The model under review builds one solid part; all positions refer to its coordinate system, in mm. Face numbers are marked on the shaded views. Give positions to 0.01 mm unless a question says otherwise; leave off trailing zeros. Order: outer loops, then holes, each group sorted by start corner. A loop starts at its lowest first (then second) coordinate and runs counter-clockwise, first axis right, second up. Notation, with made-up numbers: (-22, 20) - (25, 20) arc R35 ccw to (25, 53) - close; hole circle Ø2 at (11.25, -16.5). An arc over 180 degrees is marked (long way). Write item = value, one per line. Start each with the question number.
1. For P1, Ø1.2, axis at x = -14.5, y = -2.5, coming from the +Z side; P2, Ø9, axis at x = 13, z = 23.5, coming from the -Y side, all flat-tipped, find the tip position at first contact; note any pin that passes through.
2. Wall thickness on probe 1 along Z at (x, y) = (0, -0.7); probe 2 along X at (y, z) = (-1, 70); probe 3 along Y at (x, z) = (-16, 47): over which ranges is each line inside the solid? List them lowest first.
3. We need section A-A, the plane z = 10. Give the boundary of the cut face in (x, y), and give its area (3 significant figures).
4. We need section B-B, the plane x = 0. Give the boundary of the cut face in (y, z), and give its area (3 significant figures).
5. We need section D-D, the plane x = 14. Give the boundary of the cut face in (y, z), and give its area (3 significant figures).
6. Mouldability with a two-part tool opening along Y and no side actions: class the marked faces 1, 2 and 3 as pulls with the +Y half, pulls with the -Y half, needs draft (parallel to the pull), parting line crosses it, or undercut.
7. We need section C-C, the plane z = 60.5. Give the boundary of the cut face in (x, y), and give its area (3 significant figures).
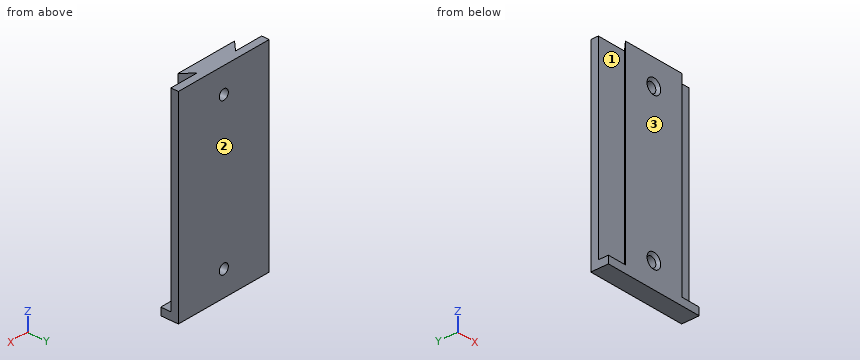
from build123d import *

# Parameters (mm, degrees)
F1_DEPTH = 80
F2_R     = 2
F3_DEPTH = 12.5
F4_SIZE  = 1
F5_W     = 40
F5_H     = 4
F6_DEPTH = 3


with BuildPart() as f1:
    # F0 (on Top) → F1 (new body)
    with BuildSketch(Plane.XY):
        Polygon((20, 1.5), (-20, 1.5), (-20, -1.5), (-8.5, -1.5), (8.5, -1.5), (20, -1.5), align=None)
        Polygon((8.5, -1.5), (-8.5, -1.5), (-12.5, -5.5), (12.5, -5.5), align=None)
    extrude(amount=F1_DEPTH)

    # F2 (on face) → F3 (cut, symmetric)
    with BuildSketch(Plane.XZ.offset(1.5)):
        with Locations((0, 70)):
            Circle(F2_R)
        with Locations((0, 10)):
            Circle(F2_R)
    extrude(amount=F3_DEPTH, both=True, mode=Mode.SUBTRACT)

    # F4
    f4_edges = [f1.edges().sort_by_distance(p)[0] for p in [
        (-2, -5.5, 70),
        (-2, -5.5, 10),
    ]]
    chamfer(f4_edges, length=F4_SIZE)

    # F5 (on Top) → F6 (join)
    with BuildSketch(Plane.XY):
        with Locations((0, -3.5)):
            Rectangle(F5_W, F5_H)
    extrude(amount=F6_DEPTH)


solid = f1.part
Model answer:
q1.P1 = 3
q1.P2 = -5.5
q2.probe_1 = 0 to 8, 12 to 68, 72 to 80
q2.probe_2 = -20 to -2, 2 to 20
q2.probe_3 = -1.5 to 1.5
q3.outline = (-20, -1.5) - (-8.5, -1.5) - (-12.5, -5.5) - (-3, -5.5) - (-2, -4.5) - (-2, 1.5) - (-20, 1.5) - close; (2, -4.5) - (3, -5.5) - (12.5, -5.5) - (8.5, -1.5) - (20, -1.5) - (20, 1.5) - (2, 1.5) - close
q3.area = 175 mm2
q4.outline = (-5.5, 0) - (1.5, 0) - (1.5, 8) - (-4.5, 8) - (-5.5, 7) - close; (-5.5, 13) - (-4.5, 12) - (1.5, 12) - (1.5, 68) - (-4.5, 68) - (-5.5, 67) - close; (-5.5, 73) - (-4.5, 72) - (1.5, 72) - (1.5, 80) - (-5.5, 80) - close
q4.area = 502 mm2
q5.outline = (-5.5, 0) - (1.5, 0) - (1.5, 80) - (-1.5, 80) - (-1.5, 3) - (-5.5, 3) - close
q5.area = 252 mm2
q6.face_1 = undercut
q6.face_2 = pulls with the +Y half
q6.face_3 = pulls with the -Y half
q7.outline = (-20, -1.5) - (-8.5, -1.5) - (-12.5, -5.5) - (12.5, -5.5) - (8.5, -1.5) - (20, -1.5) - (20, 1.5) - (-20, 1.5) - close
q7.area = 204 mm2
